Source: CAD feature listing. Evaluate the final solid. Frame: model axes, mm. Face numbers are marked on the shaded views. A direction names the side the tool comes from. Give positions to 0.01 mm unless a question says otherwise; leave off trailing zeros. Write each loop counter-clockwise with the first axis right and the second up, starting at its lowest first coordinate (ties: lowest second). Pieces come first, ordered by that corner, then holes. Notation, with made-up numbers: (-26.75, -8) - (21.25, -8) arc R24 ccw to (21.25, 24) - close; hole circle Ø11 at (-18.75, -34). An arc over 180 degrees is marked (long way). One line per question, with ' | ' between items. Start each with the question number.
(1) Draft query along X for the marked faces 6, 7, 8 and 9. Return one class per face: +X half, -X half, draft (parallel to the pull), parting line (faces both ways), or undercut.
(2) Access query for the marked faces 1, 2, 3, 4 and 5. Directions: +Z, -Z, +X, -X, +Y, -Y. A direction counts if a zero-diameter tool reaches every point of the face in a straight line with its end or side. Return the directions, or none.
(3) Section C-C, the plane x = -6.5. Return loops of the section in (y, z).
(4) Section B-B, the plane x = 1.25. Return loops of the section in (y, z), plus the area to 3 significant figures.
(5) Section A-A, the plane y = 4.5. Return loops of the section in (x, z).
(6) Ray query, line 1 (X direction, y = -9, z = 1); line 2 (X direction, y = 27, z = 7); line 3 (Y direction, x = 0.25, z = 2.25). Return the intervals inside material, ascending. Write a range as [from, to].
(7) Section D-D, the plane x = 7.5. Return loops of the section in (y, z), plus the area to 3 significant figures.
(8) Pin query (flat end, axial travel): pin 1 (3 mm diameter, centred on x = 8, z = -3.5, fed in from +Y); pin 2 (3.5 mm diameter, centred on y = 22, z = 0, fed in from +X); pin 3 (1 mm diameter, centred on x = 7.5, y = 3, fed in from +Z). Return the tip coordinate at first contact, or that it passes through.
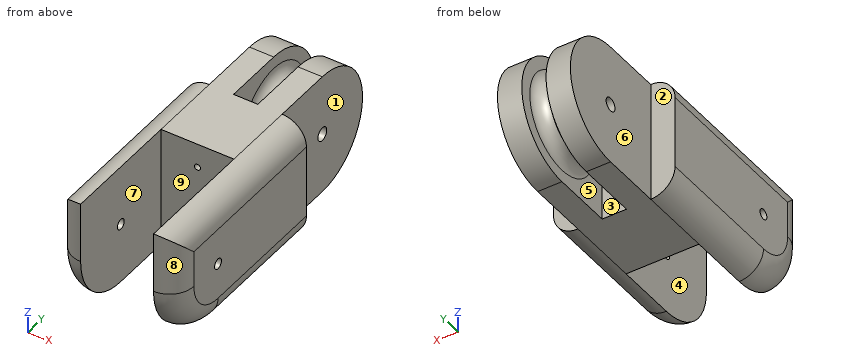
```python
from build123d import *

# Parameters (mm, degrees)
SKETCH1_W           = 20
SKETCH1_H           = 20
BOSS_EXTRUDE1_DEPTH = 12
SKETCH4_W           = 4
SKETCH4_H           = 20
BOSS_EXTRUDE2_DEPTH = 10
BOSS_EXTRUDE3_DEPTH = 4
BOSS_EXTRUDE4_START = -4
BOSS_EXTRUDE4_DEPTH = 4
SKETCH7_R           = 0.85
CUT_EXTRUDE1_DEPTH  = 31
FILLET1_R           = 4
SKETCH8_W           = 4
SKETCH8_H           = 20
BOSS_EXTRUDE5_DEPTH = 10
SKETCH9_R           = 10
BOSS_EXTRUDE6_DEPTH = 4
BOSS_EXTRUDE7_START = -4
SKETCH10_R          = 10
BOSS_EXTRUDE7_DEPTH = 4
SKETCH12_R          = 1.1
CUT_EXTRUDE2_DEPTH  = 38.148351242
SKETCH13_R          = 6
BOSS_EXTRUDE8_DEPTH = 4
SKETCH14_R          = 1.1
CUT_EXTRUDE3_DEPTH  = 4
FILLET2_R           = 2
CUT_EXTRUDE4_REACH  = 36.986
SKETCH16_R          = 0.5


with BuildPart() as part:
    # Sketch1 → Boss-Extrude1 (new body)
    with BuildSketch(Plane(origin=(0, 0, 0), x_dir=(1, 0, 0), z_dir=(0, 1, 0))):
        Rectangle(SKETCH1_W, SKETCH1_H)
    extrude(amount=BOSS_EXTRUDE1_DEPTH)

    # Sketch4 → Boss-Extrude2 (add)
    with BuildSketch(Plane.XZ):
        with Locations((-8, 0)):
            Rectangle(SKETCH4_W, SKETCH4_H)
        with Locations((8, 0)):
            Rectangle(SKETCH4_W, SKETCH4_H)
    extrude(amount=BOSS_EXTRUDE2_DEPTH)

    # Sketch5 → Boss-Extrude3 (add)
    with BuildSketch(Plane.ZY.offset(10)):
        with BuildLine():
            Line((0, -20), (10, -20))
            Line((10, -20), (10, -10))
            ThreePointArc((10, -10), (-7.071067812, -2.928932188), (0, -20))
        make_face()
    extrude(amount=-BOSS_EXTRUDE3_DEPTH)

    # Sketch6 → Boss-Extrude4 (add)
    with BuildSketch(Plane(origin=(10, 0, 0), x_dir=(0, 0, -1), z_dir=(1, 0, 0)).offset(BOSS_EXTRUDE4_START)):
        with BuildLine():
            Line((0, -20), (-10, -20))
            Line((-10, -20), (-10, -10))
            ThreePointArc((-10, -10), (7.071067812, -2.928932188), (0, -20))
        make_face()
    extrude(amount=BOSS_EXTRUDE4_DEPTH)

    # Sketch7 → Cut-Extrude1 (cut, through all)
    with BuildSketch(Plane.ZY.offset(10)):
        with Locations((0, -10)):
            Circle(SKETCH7_R)
    extrude(amount=-CUT_EXTRUDE1_DEPTH, mode=Mode.SUBTRACT)

    # Fillet1
    fillet1_edges = [part.edges().sort_by_distance(p)[0] for p in [
        (-10, -4, 10),
        (-10, -17.071067812, -7.071067812),
        (10, -4, 10),
        (10, -17.071067812, -7.071067812),
        (-10, 1, -10),
        (10, 1, -10),
        (10, -20, 5),
        (-10, -20, 5),
    ]]
    fillet(fillet1_edges, radius=FILLET1_R - 0.0001)  # a hair under: the kernel refuses the full size

    # Sketch8 → Boss-Extrude5 (add)
    with BuildSketch(Plane(origin=(0, 12, 0), x_dir=(1, 0, 0), z_dir=(0, 1, 0))):
        with Locations((4, 0)):
            Rectangle(SKETCH8_W, SKETCH8_H)
        with Locations((-4, 0)):
            Rectangle(SKETCH8_W, SKETCH8_H)
    extrude(amount=BOSS_EXTRUDE5_DEPTH)

    # Sketch9 → Boss-Extrude6 (add)
    with BuildSketch(Plane(origin=(6, 0, 0), x_dir=(0, 0, -1), z_dir=(1, 0, 0))):
        with Locations((0, 22)):
            Circle(SKETCH9_R)
    extrude(amount=-BOSS_EXTRUDE6_DEPTH)

    # Sketch10 → Boss-Extrude7 (add)
    with BuildSketch(Plane.ZY.offset(6).offset(BOSS_EXTRUDE7_START)):
        with Locations((0, 22)):
            Circle(SKETCH10_R)
    extrude(amount=BOSS_EXTRUDE7_DEPTH)

    # Sketch12 → Cut-Extrude2 (cut, through all)
    with BuildSketch(Plane.ZY.offset(6)):
        with Locations((0, 22)):
            Circle(SKETCH12_R)
    extrude(amount=-CUT_EXTRUDE2_DEPTH, mode=Mode.SUBTRACT)

    # Sketch13 → Boss-Extrude8 (add)
    with BuildSketch(Plane(origin=(-2, 0, 0), x_dir=(0, 0, -1), z_dir=(1, 0, 0))):
        with Locations(Location((0, 22, 0), (0, 0, 180))):
            Circle(SKETCH13_R)
    extrude(amount=BOSS_EXTRUDE8_DEPTH)

    # Sketch14 → Cut-Extrude3 (cut)
    with BuildSketch(Plane(origin=(-2, 0, 0), x_dir=(0, 0, -1), z_dir=(1, 0, 0))):
        with Locations(Location((0, 22, 0), (0, 0, 180))):
            Circle(SKETCH14_R)
    extrude(amount=CUT_EXTRUDE3_DEPTH, mode=Mode.SUBTRACT)

    # Fillet2
    fillet2_edges = [part.edges().sort_by_distance(p)[0] for p in [
        (-2, 22, -6),
        (2, 22, -6),
    ]]
    fillet(fillet2_edges, radius=FILLET2_R - 0.0001)  # a hair under: the kernel refuses the full size

    # Sketch16 → Cut-Extrude4 (cut, up to next)
    with BuildSketch(Plane.XZ, mode=Mode.PRIVATE) as cut_extrude4_sk1:
        with Locations(Location((0, -6, 0), (0, 0, 270))):
            Circle(SKETCH16_R)
    cut_extrude4_tool1 = extrude(cut_extrude4_sk1.sketch, amount=-CUT_EXTRUDE4_REACH, mode=Mode.PRIVATE) & part.part
    # Sketch16 → Cut-Extrude4 (cut, up to next)
    with BuildSketch(Plane.XZ, mode=Mode.PRIVATE) as cut_extrude4_sk2:
        with Locations(Location((0, 6, 0), (0, 0, 90))):
            Circle(SKETCH16_R)
    cut_extrude4_tool2 = extrude(cut_extrude4_sk2.sketch, amount=-CUT_EXTRUDE4_REACH, mode=Mode.PRIVATE) & part.part
    add(cut_extrude4_tool1.solids().sort_by_distance((0, 0, -6))[0], mode=Mode.SUBTRACT)
    add(cut_extrude4_tool2.solids().sort_by_distance((0, 0, 6))[0], mode=Mode.SUBTRACT)


solid = part.part
```
Check sheet entries:
1) face 6: -X half | face 7: undercut | face 8: +X half | face 9: undercut
2) face 1: +Z, -Z, +X, +Y | face 2: +Z, -Z, -X, +Y | face 3: +Z, -Z | face 4: +Z, -Z, -Y | face 5: none
3) outline: (-19.97, 0) arc R9.97 ccw to (-10, -9.97) - (12, -9.97) - (12, 9.97) - (-19.97, 9.97) - close; hole circle Ø1.7 at (-10, 0)
4) outline: (0, -10) - (12, -10) - (12, 10) - (0, 10) - close; circle Ø12.88 at (22, 0); hole circle Ø2.2 at (22, 0) | area: 366 mm²
5) outline: (-10, -6) arc R4 ccw to (-6, -10) - (6, -10) arc R4 ccw to (10, -6) - (10, 6) arc R4 ccw to (6, 10) - (-6, 10) arc R4 ccw to (-10, 6) - close; hole circle Ø1 at (0, -6); hole circle Ø1 at (0, 6)
6) line 1: [-10, -6], [6, 10] | line 2: [-6, -2], [2, 6] | line 3: [0, 12], [16.42, 27.58]
7) outline: (-19.71, 0) arc R9.71 ccw to (-10, -9.71) - (12, -9.71) - (12, 9.71) - (-19.71, 9.71) - close; hole circle Ø1.7 at (-10, 0) | area: 593 mm²
8) pin 1: y = 12 | pin 2: x = 6 | pin 3: z = 9.87
